from build123d import *

# Parameters (mm, degrees)
F1_DEPTH = 3.175
F2_R     = 0.9525
F3_DEPTH = 6.35


# Not quite as in the source:
# - a length typed as a fraction of an inch, garbled in the dataset ("3 / 203.2 mm" for 3/8 in), is restored


with BuildPart() as f1:
    # F0 (on Top) → F1 (new body)
    with BuildSketch(Plane.XY):
        with BuildLine():
            Line((0, 4.3302561211), (0, 0))
            Line((0, 0), (12.7, 0))
            Line((12.7, 0), (15.24, 2.54))
            Line((15.24, 2.54), (21.6802561211, 8.9802561211))
            Line((21.6802561211, 8.9802561211), (21.6802561211, 21.6802561211))
            Line((21.6802561211, 21.6802561211), (12.7, 30.6605122421))
            Line((12.7, 30.6605122421), (0, 30.6605122421))
            Line((0, 30.6605122421), (-2.54, 28.1205122421))
            Line((-2.54, 28.1205122421), (-8.9802561211, 21.6802561211))
            Line((-8.9802561211, 21.6802561211), (-3.5386407003, 10.5120837393))
            ThreePointArc((-3.5386407003, 10.5120837393), (12.1809563452, 24.657632392), (6.35, 4.3302561211))
            Line((6.35, 4.3302561211), (0, 4.3302561211))
        make_face()
    extrude(amount=F1_DEPTH)

    # F2 (on face) → F3 (join)
    with BuildSketch(Plane(origin=(6.35, -6.35, 0), x_dir=(0.7071067812, 0.7071067812, 0), z_dir=(0.7071067812, -0.7071067812, 0))):
        with Locations((15.3302561211, 1.5875)):
            Circle(F2_R)
    extrude(amount=F3_DEPTH)


solid = f1.part
For this review, take the finished solid that the model builds, in its own axes (mm). A direction names the side the tool comes from. Coordinates: 2 decimals unless noted, no trailing zeros. Write each loop counter-clockwise with the first axis right and the second up, starting at its lowest first coordinate (ties: lowest second). Pieces come first, ordered by that corner, then holes. Notation, with made-up numbers: (-4.5, 34) -> (1.5, 34) arc R6 cw to (1.5, 40) -> close; hole circle Ø2 at (45.5, 20). An arc over 180 degrees is marked (long way). Write each question's results on one line, items separated by ' | '. Start each with the question number.
1) Consider section A-A (x = 14.5). Write out the cut boundary in (y, z) (3 decimals), plus the area to 3 significant figures.
2) The part is to be moulded in two halves that separate along Y. For faces 6 (the face through (6, 30.661, 2)), 7 (the face through (-6.298, 16.174, 1.565)), 8 (the face through (18.907, 1.78, 2.231)), say which applies: +Y half, -Y half, draft (parallel to the pull), parting line (faces both ways), or undercut.
3) For faces 1 (the face through (6, 0, 2)), 2 (the face through (13.1, 24.5, 3.175)), 3 (the face through (21.68, 15, 2)), 4 (the face through (3, 4.33, 2)), 5 (the face through (13.1, 24.5, 0)), list the 3-axis set-ups (+Z, -Z, +X, -X, +Y, -Y) from which the entire face can be reached by the end or side of a thin tool; tool diameter is ignored.
4) Consider section D-D (y = 6). Write out the cut boundary in (x, z) (3 decimals).
5) Consider section B-B (y = 21). Write out the cut boundary in (x, z) (3 decimals).
6) Wall thickness on L1, parallel to Y at x = 6.5, z = 2.65; L2, parallel to Y at x = 7.5, z = 0.75; L3, parallel to X at y = 1, z = 0.95: over which ranges is each line inside the solid? List them lowest first. Write a range as [from, to].
7) Insertion check: pin 1 (1.6 mm diameter, centred on y = 2.5, z = 1, fed in from -X); pin 2 (3 mm diameter, centred on x = 3, y = 25, fed in from +Z) (3 decimals); pin 3 (1.6 mm diameter, centred on y = 15, z = 2, fed in from +X); pin 4 (6 mm diameter, centred on x = 12.5, y = 12.5, fed in from -Z). Each pin has a flat end and moves straight along its axis. Give the tip position at first contact, or say it passes through.
8) Consider section C-C (x = -3). Write out the cut boundary in (y, z) (3 decimals).
Geometry says:
1) outline: (1.8, 0) -> (7.943, 0) -> (7.943, 3.175) -> (1.8, 3.175) -> close; (22.718, 0) -> (28.861, 0) -> (28.861, 3.175) -> (22.718, 3.175) -> close | area: 39.0 mm^2
2) face 6: +Y half | face 7: -Y half | face 8: undercut
3) face 1: +Z, -Z, -X, -Y | face 2: +Z, +X, -X, +Y, -Y | face 3: +Z, -Z, +X, +Y | face 4: +Z, -Z, -X | face 5: -Z, +X, -X, +Y, -Y
4) outline: (12.176, 0) -> (18.7, 0) -> (18.7, 3.175) -> (12.176, 3.175) -> close
5) outline: (-8.649, 0) -> (-3.076, 0) -> (-3.076, 3.175) -> (-8.649, 3.175) -> close; (15.776, 0) -> (21.68, 0) -> (21.68, 3.175) -> (15.776, 3.175) -> close
6) L1: [0, 4.33], [26.33, 30.66] | L2: [0, 4.39], [26.27, 30.66] | L3: [0, 13.7], [19.68, 21.68]
7) pin 1: x = 0 | pin 2: z = 3.175 | pin 3: x = 21.68 | pin 4: through
8) outline: (21.125, 0) -> (27.661, 0) -> (27.661, 3.175) -> (21.125, 3.175) -> close
